Could you check a few things on this model? Use its own coordinates, in mm. A direction names the side the tool comes from. Coordinates: 2 decimals unless noted, no trailing zeros. Write each loop counter-clockwise with the first axis right and the second up, starting at its lowest first coordinate (ties: lowest second). Pieces come first, ordered by that corner, then holes. Notation, with made-up numbers: (69, 58) - (86, 58) arc R18 ccw to (86, 78) - close; hole circle Ø3 at (34.25, -36). An arc over 180 degrees is marked (long way). Write item = value, one per line. Start each with the question number.
```python
from build123d import *

# Parameters (mm, degrees)
SKETCH1_W                = 3.175
SKETCH1_H                = 19.4818
CUT_EXTRUDE1_START       = -3.302
CUT_EXTRUDE1_DEPTH       = 3.302
CUT_EXTRUDE2_START       = -3.302
CUT_EXTRUDE2_DEPTH       = 3.302
M3_CLEARANCE_HOLE1_D     = 3.40106
M3_CLEARANCE_HOLE1_DEPTH = 11.684
CHAMFER1_SIZE            = 0.38227


with BuildPart() as part:
    # Sketch1 → Revolve1 (revolve)
    with BuildSketch(Plane(origin=(0, 0, 0), x_dir=(-1, 0, 0), z_dir=(0, 0, -1)), mode=Mode.PRIVATE) as revolve1_sk:
        with Locations((-1.5875, 9.7409)):
            Rectangle(SKETCH1_W, SKETCH1_H)
    revolve(revolve1_sk.sketch.rotate(Axis((0, 0, 0), (0, 1, 0)), 270), axis=Axis((0, 0, 0), (0, 1, 0)))

    # Sketch2 → Cut-Extrude1 (cut)
    with BuildSketch(Plane(origin=(0, 19.4818, 0), x_dir=(-1, 0, 0), z_dir=(0, 1, 0)).offset(CUT_EXTRUDE1_START)):
        with BuildLine():
            Line((2.794, 1.508041445), (2.794, -1.508041445))
            ThreePointArc((2.794, -1.508041445), (3.175, 0), (2.794, 1.508041445))
        make_face()
    extrude(amount=CUT_EXTRUDE1_DEPTH, mode=Mode.SUBTRACT)

    # Sketch3 → Cut-Extrude2 (cut)
    with BuildSketch(Plane(origin=(0, 19.4818, 0), x_dir=(-1, 0, 0), z_dir=(0, 1, 0)).offset(CUT_EXTRUDE2_START)):
        with BuildLine():
            Line((-2.794, -1.508041445), (-2.794, 1.508041445))
            ThreePointArc((-2.794, 1.508041445), (-3.175, 0), (-2.794, -1.508041445))
        make_face()
    extrude(amount=CUT_EXTRUDE2_DEPTH, mode=Mode.SUBTRACT)

    # M3 Clearance Hole1
    with Locations(Plane(origin=(0, 19.4818, 0), x_dir=(1, 0, 0), z_dir=(0, 1, 0))):
        with Locations((0, 0)):
            Hole(M3_CLEARANCE_HOLE1_D / 2, depth=M3_CLEARANCE_HOLE1_DEPTH)

    # Chamfer1
    chamfer1_edges = [part.edges().sort_by_distance(p)[0] for p in [
        (1.70053, 19.4818, 0),
    ]]
    chamfer(chamfer1_edges, length=CHAMFER1_SIZE)


solid = part.part
```
1) Suppose I cut it at B-B on z = 0. Please give me the cut outline in (x, y) (3 decimals), plus the area to 3 significant figures.
2) Which directions (+Z, -Z, +X, -X, +Y, -Y) give clear straight access to the entire face, cutting with the end or side of a thin tool? Please do faces 1 (the flat face through (2.794, 18, 0)), 2 (the flat face through (0, 0, 0)), 3 (the flat face through (0, 7.798, 0)).
3) Suppose I cut it at C-C on y = 14. Please give me the cut outline in (x, z) (3 decimals), plus the area to 3 significant figures.
4) For P1, Ø3.5, axis at y = 18.5, z = -0.5, coming from the +X side; P2, Ø1.5, axis at y = 13, z = 1, coming from the -X side; P3, Ø2, axis at x = 0, z = 0, coming from the +Y side, each with a flat end and sliding along its axis, tell me the tip position at first contact or that it passes through.
5) Thinking about a two-plate mould opening in Z: for faces 4 (the cylindrical face through (0.37, 13.37, 1.66)), 5 (the flat face through (-2.794, 18, 0)), 6 (the cylindrical face through (3.15, 9.88, -0.41)), which applies, +Z half, -Z half, draft (parallel to the pull), parting line (faces both ways), or undercut?
6) Suppose I cut it at D-D on y = 7. Please give me the cut outline in (x, z) (3 decimals), plus the area to 3 significant figures.
7) Suppose I cut it at A-A on x = 0. Please give me the cut outline in (y, z) (3 decimals), plus the area to 3 significant figures.
8) If I drill on probe 1 along Z at (x, y) = (0, 14.5) (3 decimals); probe 2 along X at (y, z) = (17, 0); probe 3 along Y at (x, z) = (-1.5, 0.25), over which ranges is the centre line in solid material (lowest first)? Write a range as [from, to].
Reply:
q1.outline = (-3.175, 0) - (3.175, 0) - (3.175, 16.18) - (2.794, 16.18) - (2.794, 19.482) - (2.083, 19.482) - (1.701, 19.1) - (1.701, 7.798) - (-1.701, 7.798) - (-1.701, 19.1) - (-2.083, 19.482) - (-2.794, 19.482) - (-2.794, 16.18) - (-3.175, 16.18) - close
q1.area = 81.3 mm^2
q2.face_1 = +Z, -Z, +X, +Y
q2.face_2 = +Z, -Z, +X, -X, -Y
q2.face_3 = +Y
q3.outline = circle Ø6.35 at (0, 0); hole circle Ø3.401 at (0, 0)
q3.area = 22.6 mm^2
q4.P1 = 2.79
q4.P2 = -3.17
q4.P3 = 7.8
q5.face_4 = undercut
q5.face_5 = draft
q5.face_6 = parting line
q6.outline = circle Ø6.35 at (0, 0)
q6.area = 31.7 mm^2
q7.outline = (0, -3.175) - (19.482, -3.175) - (19.482, -2.083) - (19.1, -1.701) - (7.798, -1.701) - (7.798, 1.701) - (19.1, 1.701) - (19.482, 2.083) - (19.482, 3.175) - (0, 3.175) - close
q7.area = 83.8 mm^2
q8.probe_1 = [-3.175, -1.701], [1.701, 3.175]
q8.probe_2 = [-2.79, -1.7], [1.7, 2.79]
q8.probe_3 = [0, 7.8]
